Can you work these out from the model? Positions are in its coordinate system, mm. Face numbers are marked on the shaded views. A direction names the side the tool comes from. Round coordinates to 2 decimals unless told otherwise and drop trailing zeros. Loops run counter-clockwise (first coordinate to the right, second up) from the corner with the lowest first, then second, coordinate; pieces in that order, holes last. Notation, with made-up numbers: (8, 55) - (27, 55) arc R13 cw to (27, 68) - close; hole circle Ø11 at (81.5, 88.25). An arc over 180 degrees is marked (long way). Answer as CSV lines item,"result".
```python
from build123d import *

# Parameters (mm, degrees)
BASE_FLANGE1_DEPTH = 20
SKETCH6_R          = 2.65
CUT_EXTRUDE1_DEPTH = 10
SKETCH7_R          = 1.65
CUT_EXTRUDE2_DEPTH = 10


# Sheet-metal steps are written as plain solids
with BuildPart() as part:
    # Sketch1 → Base-Flange1 (new body)
    with BuildSketch(Plane.XY):
        with BuildLine():
            Line((-15.568720379, 20), (-6.568720379, 20))
            ThreePointArc((-6.568720379, 20), (-2.326079692, 18.242640687), (-0.568720379, 14))
            Line((-0.568720379, 14), (-0.568720379, 3))
            ThreePointArc((-0.568720379, 3), (0.309959277, 0.878679656), (2.431279621, 0))
            Line((2.431279621, 0), (14.431279621, 0))
            Line((14.431279621, 0), (14.431279621, -3))
            Line((14.431279621, -3), (2.431279621, -3))
            ThreePointArc((2.431279621, -3), (-1.811361066, -1.242640687), (-3.568720379, 3))
            Line((-3.568720379, 3), (-3.568720379, 14))
            ThreePointArc((-3.568720379, 14), (-4.447400036, 16.121320344), (-6.568720379, 17))
            Line((-6.568720379, 17), (-15.568720379, 17))
            Line((-15.568720379, 17), (-15.568720379, 20))
        make_face()
    extrude(amount=BASE_FLANGE1_DEPTH)

    # Sketch6 → Cut-Extrude1 (cut)
    with BuildSketch(Plane(origin=(0, 20, 0), x_dir=(1, 0, 0), z_dir=(0, 1, 0))):
        with Locations(Location((-11.068720379, -10, 0), (0, 0, 270))):
            Circle(SKETCH6_R)
    extrude(amount=-CUT_EXTRUDE1_DEPTH, mode=Mode.SUBTRACT)

    # Sketch7 → Cut-Extrude2 (cut)
    with BuildSketch(Plane(origin=(0, 0, 0), x_dir=(1, 0, 0), z_dir=(0, 1, 0))):
        with Locations(Location((8.431279621, -10, 0), (0, 0, 270))):
            Circle(SKETCH7_R)
    extrude(amount=-CUT_EXTRUDE2_DEPTH, mode=Mode.SUBTRACT)


solid = part.part
```
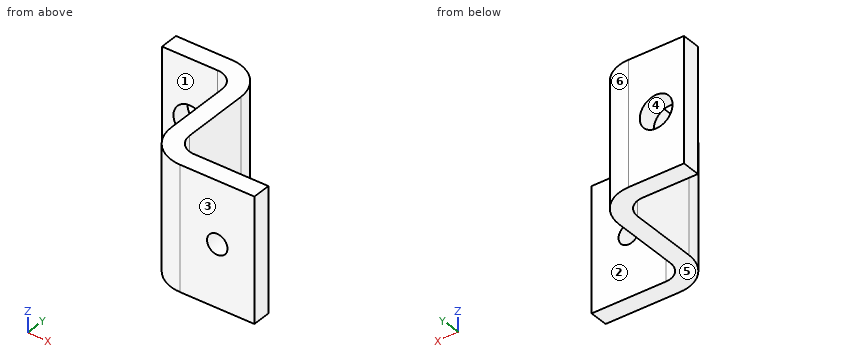
Q1. We'd pull the mould along Z, two halves only. Please class the marked faces 4, 5 and 6: pulls with the +Z half, pulls with the -Z half, needs draft (parallel to the pull), parting line crosses it, or undercut.
Checks:
face 4,"undercut"
face 5,"pulls with the -Z half"
face 6,"needs draft"
Q2. Imagine slicing it at D-D (y = 8.25). Write out the boundary of the cut face in (x, z), then the cut area to 3 significant figures.
Checks:
outline,"(-3.57, 0) - (-0.57, 0) - (-0.57, 20) - (-3.57, 20) - close"
area,"60.0 mm²"
Q3. On a 3-axis mill with a long thin cutter (end or side, diameter ignored), from which of +Z, -Z, +X, -X, +Y, -Y can I reach the whole of each face in a straight line? I mean the marked faces 1, 2 and 3. Say none if no direction works.
Checks:
face 1,"+Z, -Z, -X, -Y"
face 2,"+Z, -Z, +X, +Y"
face 3,"+Z, -Z, +X, -X, -Y"
Q4. Imagine slicing it at C-C (x = 3.75). Write out the boundary of the cut face in (y, z), then the cut area to 3 significant figures.
Checks:
outline,"(-3, 0) - (0, 0) - (0, 20) - (-3, 20) - close"
area,"60.0 mm²"
Q5. I'm going to push flat-ended pins straight in: pin 1 Ø9 at (y, z) = (9.5, 10.5) entering from -X; pin 2 Ø1.5 at (y, z) = (12, 15.5) entering from +X; pin 3 Ø10 at (x, z) = (-11.5, 18) entering from -Y. Where does each tip first touch, or does it pass through?
Checks:
pin 1,"x = -3.57"
pin 2,"x = -0.57"
pin 3,"y = 17"
Q6. Imagine slicing it at B-B (z = 15). Write out the boundary of the cut face in (x, y).
Checks:
outline,"(-15.57, 17) - (-6.57, 17) arc R3 cw to (-3.57, 14) - (-3.57, 3) arc R6 ccw to (2.43, -3) - (14.43, -3) - (14.43, 0) - (2.43, 0) arc R3 cw to (-0.57, 3) - (-0.57, 14) arc R6 ccw to (-6.57, 20) - (-15.57, 20) - close"
Q7. If I drill on line 1 along X through (y, z) = (3.75, 11); line 2 along X through (y, z) = (17.95, 10); line 3 along X through (y, z) = (-1.75, 10), over which ranges is the centre line in solid material (lowest first)? Write a range as [from, to].
Checks:
line 1,"[-3.57, -0.57]"
line 2,"[-15.57, -13.72], [-8.42, -2.05]"
line 3,"[-1.23, 6.78], [10.08, 14.43]"
Q8. Imagine slicing it at A-A (z = 10). Write out the boundary of the cut face in (x, y), then the cut area to 3 significant figures.
Checks:
outline,"(-15.57, 17) - (-13.72, 17) - (-13.72, 20) - (-15.57, 20) - close; (-8.42, 17) - (-6.57, 17) arc R3 cw to (-3.57, 14) - (-3.57, 3) arc R6 ccw to (2.43, -3) - (6.78, -3) - (6.78, 0) - (2.43, 0) arc R3 cw to (-0.57, 3) - (-0.57, 14) arc R6 ccw to (-6.57, 20) - (-8.42, 20) - close; (10.08, -3) - (14.43, -3) - (14.43, 0) - (10.08, 0) - close"
area,"113 mm²"
